```python
from build123d import *

# Parameters (mm, degrees)
ESQUISSE1_W        = 20
ESQUISSE1_H        = 41
BOSS_EXTRU_1_DEPTH = 10
CONG_1_R           = 10
CONG_2_R           = 10


with BuildPart() as part:
    # Esquisse1 → Boss.-Extru.1 (new body)
    with BuildSketch(Plane.XY):
        with BuildLine():
            Line((-7.391944515, 10.850266565), (19.223939946, 10.850266565))
            ThreePointArc((19.223939946, 10.850266565), (32.688147419, -68.35721731), (-14.757789944, -133.195426819))
            ThreePointArc((-14.757789944, -133.195426819), (0.583223132, -89.904856397), (-7.391944515, -44.674149232))
            Line((-7.391944515, -44.674149232), (-7.391944515, 10.850266565))
        make_face()
        with Locations((10, -20.5)):
            Rectangle(ESQUISSE1_W, ESQUISSE1_H, mode=Mode.SUBTRACT)
    extrude(amount=BOSS_EXTRU_1_DEPTH)

    # Congé1
    cong_1_edges = [part.edges().sort_by_distance(p)[0] for p in [
        (19.223939946, 10.850266565, 5),
    ]]
    fillet(cong_1_edges, radius=CONG_1_R)

    # Congé2
    cong_2_edges = [part.edges().sort_by_distance(p)[0] for p in [
        (-7.391944515, -44.674149232, 5),
        (-7.391944515, 10.850266565, 5),
    ]]
    fillet(cong_2_edges, radius=CONG_2_R)


solid = part.part
```
Read the model definition and answer for the solid it produces. Units are mm, in the model's axes. A direction names the side the tool comes from. Coordinates: 2 decimals unless noted, no trailing zeros. Loops run counter-clockwise (first coordinate to the right, second up) from the corner with the lowest first, then second, coordinate; pieces in that order, holes last. Notation, with made-up numbers: (-29.75, 84.5) -> (-21.75, 84.5) arc R13 cw to (-21.75, 91.5) -> close; hole circle Ø1 at (27, 40.5). An arc over 180 degrees is marked (long way). Return JSON: item names as keys, results as strings.
Item 1: Find section C-C (y = -30.5). Determine the outline of the cut face in (x, z).
Answers:
{"outline": "(-7.39, 0) -> (0, 0) -> (0, 10) -> (-7.39, 10) -> close; (20, 0) -> (34.47, 0) -> (34.47, 10) -> (20, 10) -> close"}
Item 2: Find section B-B (x = 6.5). Determine the outline of the cut face in (y, z), plus the area to 3 significant figures.
Answers:
{"outline": "(-116.32, 0) -> (-41, 0) -> (-41, 10) -> (-116.32, 10) -> close; (0, 0) -> (10.85, 0) -> (10.85, 10) -> (0, 10) -> close", "area": "862 mm2"}
Item 3: For faces 1 (the flat face through (8, 10.85, 5)), 2 (the flat face through (-7.392, -21, 5)), 3 (the flat face through (0, -21, 5)), determine the directions among +Z, -Z, +X, -X, +Y, -Y from which every point of the face is accessible in a straight line to the end or side of a thin tool.
Answers:
{"face 1": "+Z, -Z, +X, -X, +Y", "face 2": "+Z, -Z, -X, +Y", "face 3": "+Z, -Z"}
Item 4: Find section D-D (y = -92). Determine the outline of the cut face in (x, z), plus the area to 3 significant figures.
Answers:
{"outline": "(0.38, 0) -> (23.95, 0) -> (23.95, 10) -> (0.38, 10) -> close", "area": "236 mm2"}
Item 5: For a pull along Y with two mould halves and no side action, classify faces 4 (the cylindrical face through (-4.385, 7.999, 5.07)), 5 (the cylindrical face through (-7.189, -44.546, 5.07)), 6 (the flat face through (11, -44, 10)), 7 (the flat face through (20, -21, 5)) as +Y half, -Y half, draft (parallel to the pull), parting line (faces both ways), or undercut.
Answers:
{"face 4": "+Y half", "face 5": "undercut", "face 6": "draft", "face 7": "undercut"}
Item 6: Find the intervals of material crossed by probe 1 along X at (y, z) = (-40, 6.75); probe 2 along X at (y, z) = (-26, 4.5); probe 3 along Y at (x, z) = (18.5, 0.5), in increasing order.
Answers:
{"probe 1": "x = -7.39 to 0, 20 to 35.34", "probe 2": "x = -7.39 to 0, 20 to 33.74", "probe 3": "y = -101.32 to -41, 0 to 9.55"}
Item 7: Flat-ended cylindrical pins translate along their axes: P1, Ø2, axis at y = -63.5, z = 7, coming from the -X side; P2, Ø2, axis at y = -95.5, z = 1.5, coming from the -X side; P3, Ø10, axis at x = 26, y = -36, coming from the -Z side; P4, Ø3, axis at x = 8, z = 4, coming from the -Y side. Find the tip coordinate at first contact, or state that the pin passes through.
Answers:
{"P1": "stops at x = -1.34", "P2": "stops at x = -0.21", "P3": "stops at z = 0", "P4": "stops at y = -116.32"}
Item 8: Find section A-A (z = 7.75). Determine the outline of the cut face in (x, y).
Answers:
{"outline": "(-14.76, -133.2) arc R103.15 ccw to (22.29, 5.74) arc R10 ccw to (13.56, 10.85) -> (2.61, 10.85) arc R10 ccw to (-7.39, 0.85) -> (-7.39, -42.54) arc R10 ccw to (-6.56, -46.52) arc R90.16 cw to start; hole (0, -41) -> (20, -41) -> (20, 0) -> (0, 0) -> close"}
